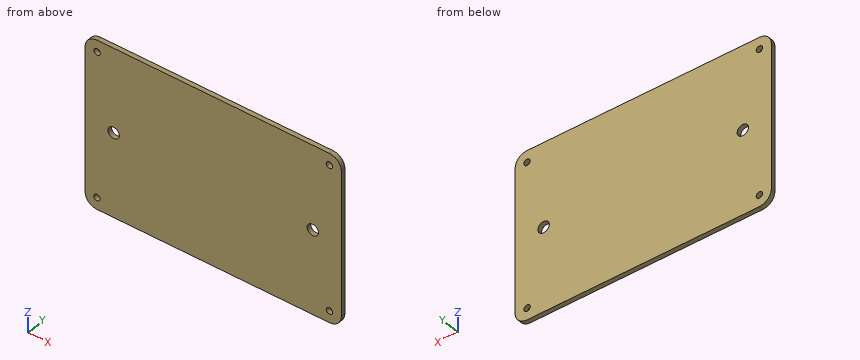
```python
from build123d import *

# Parameters (mm, degrees)
SKETCH2_R           = 1.1303
BOSS_EXTRUDE3_DEPTH = 1.59
SKETCH3_R           = 2
CUT_EXTRUDE1_DEPTH  = 1.59


with BuildPart() as part:
    # Sketch2 → Boss-Extrude3 (new body)
    with BuildSketch(Plane(origin=(0, 0, 0), x_dir=(1, 0, 0), z_dir=(0, 1, 0))):
        with BuildLine():
            Line((-45, 25.825), (-45, -25.825))
            ThreePointArc((-45, -25.825), (-43.777170811, -28.777170811), (-40.825, -30))
            Line((-40.825, -30), (40.825, -30))
            ThreePointArc((40.825, -30), (43.777170811, -28.777170811), (45, -25.825))
            Line((45, -25.825), (45, 25.825))
            ThreePointArc((45, 25.825), (43.777170811, 28.777170811), (40.825, 30))
            Line((40.825, 30), (-40.825, 30))
            ThreePointArc((-40.825, 30), (-43.777170811, 28.777170811), (-45, 25.825))
        make_face()
        with Locations(Location((40.825, 25.825, 0), (0, 0, 90))):
            Circle(SKETCH2_R, mode=Mode.SUBTRACT)
        with Locations(Location((-40.825, 25.825, 0), (0, 0, 90))):
            Circle(SKETCH2_R, mode=Mode.SUBTRACT)
        with Locations(Location((-40.825, -25.825, 0), (0, 0, 90))):
            Circle(SKETCH2_R, mode=Mode.SUBTRACT)
        with Locations(Location((40.825, -25.825, 0), (0, 0, 90))):
            Circle(SKETCH2_R, mode=Mode.SUBTRACT)
    extrude(amount=BOSS_EXTRUDE3_DEPTH)

    # Sketch3 → Cut-Extrude1 (cut)
    with BuildSketch(Plane.XZ):
        with Locations(Location((-35, 0, 0), (0, 0, 270))):
            Circle(SKETCH3_R)
        with Locations(Location((35, 0, 0), (0, 0, 270))):
            Circle(SKETCH3_R)
    extrude(amount=-CUT_EXTRUDE1_DEPTH, mode=Mode.SUBTRACT)


solid = part.part
```
Check sheet for the modelled part. Datum: model origin and axes. Units: mm. Give positions to 0.01 mm unless a question says otherwise; leave off trailing zeros. Order: outer loops, then holes, each group sorted by start corner. A loop starts at its lowest first (then second) coordinate and runs counter-clockwise, first axis right, second up. Notation, with made-up numbers: (-8, 44.5) -> (22, 44.5) arc R5 cw to (22, 51.5) -> close; hole circle Ø3 at (-7, 77). An arc over 180 degrees is marked (long way). Return JSON: item names as keys, results as strings.
1. Go/stop test with a flat-tipped pin: P1, Ø1.4, axis at x = 40.825, z = 25.825, coming from the -Y side. Record where the tip stops, or that it passes through.
From the geometry:
{"P1": "through"}
2. Cross-section at A-A, the plane x = 35. Record the cut outline in (y, z), plus the area to 3 significant figures.
From the geometry:
{"outline": "(0, -30) -> (1.59, -30) -> (1.59, -2) -> (0, -2) -> close; (0, 2) -> (1.59, 2) -> (1.59, 30) -> (0, 30) -> close", "area": "89.0 mm^2"}
3. Material ranges on probe 1 along X at (y, z) = (0.65, 0); probe 2 along X at (y, z) = (0.55, -26.5); probe 3 along X at (y, z) = (1.15, -27.5), recorded low to high. Write a range as [from, to].
From the geometry:
{"probe 1": "[-45, -37], [-33, 33], [37, 45]", "probe 2": "[-44.95, -41.73], [-39.92, 39.92], [41.73, 44.95]", "probe 3": "[-44.65, 44.65]"}
4. Cross-section at B-B, the plane z = 0. Record the cut outline in (x, y), plus the area to 3 significant figures.
From the geometry:
{"outline": "(-45, 0) -> (-37, 0) -> (-37, 1.59) -> (-45, 1.59) -> close; (-33, 0) -> (33, 0) -> (33, 1.59) -> (-33, 1.59) -> close; (37, 0) -> (45, 0) -> (45, 1.59) -> (37, 1.59) -> close", "area": "130 mm^2"}
